The figure shows three views and two pictorial views of one solid part (mm, origin at its lowest corner). Answer the questions. Give positions to 0.01 mm unless a question says otherwise; leave off trailing zeros. Order: outer loops, then holes, each group sorted by start corner. A loop starts at its lowest first (then second) coordinate and runs counter-clockwise, first axis right, second up. Notation, with made-up numbers: (20, 10) - (59, 10) arc R13 ccw to (59, 17) - close; hole circle Ø11 at (45.5, 6). An arc over 180 degrees is marked (long way). Answer as a JSON object with one key per item and string values. Group by question number.
Q1. Consider line 1 (Z direction, x = 4.5, y = 7.8); line 2 (X direction, y = 8.35, z = 5); line 3 (X direction, y = 3.75, z = 117). Determine where each line is inside the solid, lowest interval first.
Q2. A cutting plane is placed at B-B, the plane y = 5.25. Give the vertices of the cut face in (x, z), and give its area (3 significant figures).
Q3. A cutting plane is placed at D-D, the plane z = 5. Give the vertices of the cut face in (x, y), and give its area (3 significant figures).
Q4. A cutting plane is placed at A-A, the plane x = 4.5. Count the separate pieces of the cut face and the enclosed holes in it, and give its area (3 significant figures).
Q5. The mould has two halves that part along Y. Classify the marked faces 1 and 2: released by +Y, released by -Y, zero draft, split by the parting line, or undercut.
Q6. A cutting plane is placed at C-C, the plane z = 95. Give the vertices of the cut face in (x, y), and give its area (3 significant figures).
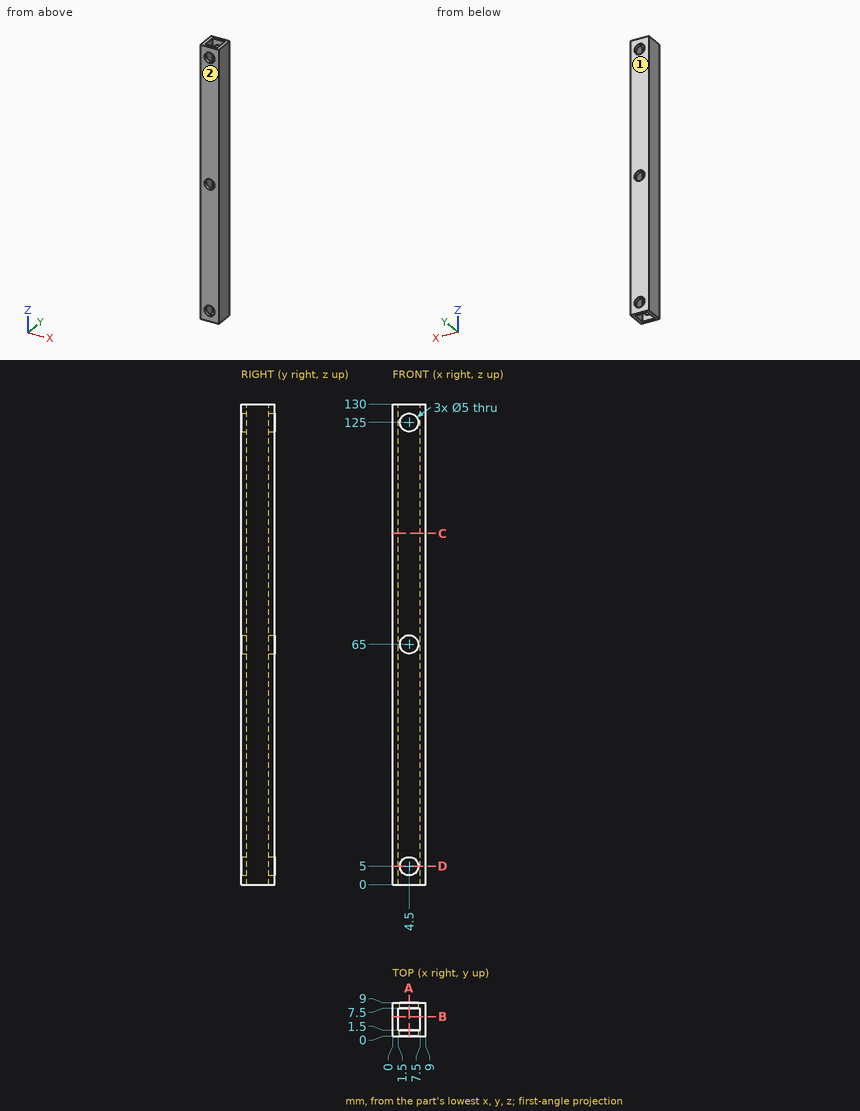
Reply:
{
 "1": {"line 1": "z = 0 to 2.5, 7.5 to 62.5, 67.5 to 122.5, 127.5 to 130", "line 2": "x = 0 to 2, 7 to 9", "line 3": "x = 0 to 1.5, 7.5 to 9"},
 "2": {"outline": "(0, 0) - (1.5, 0) - (1.5, 130) - (0, 130) - close; (7.5, 0) - (9, 0) - (9, 130) - (7.5, 130) - close", "area": "390 mm^2"},
 "3": {"outline": "(0, 0) - (2, 0) - (2, 1.5) - (1.5, 1.5) - (1.5, 7.5) - (2, 7.5) - (2, 9) - (0, 9) - close; (7, 0) - (9, 0) - (9, 9) - (7, 9) - (7, 7.5) - (7.5, 7.5) - (7.5, 1.5) - (7, 1.5) - close", "area": "30.0 mm^2"},
 "4": {"separate pieces": "8", "enclosed holes": "0", "area": "345 mm^2"},
 "5": {"face 1": "released by +Y", "face 2": "released by -Y"},
 "6": {"outline": "(0, 0) - (9, 0) - (9, 9) - (0, 9) - close; hole (1.5, 1.5) - (7.5, 1.5) - (7.5, 7.5) - (1.5, 7.5) - close", "area": "45.0 mm^2"}
}
